The model under review builds one solid part; all positions refer to its coordinate system, in mm. A direction names the side the tool comes from. Coordinates: 2 decimals unless noted, no trailing zeros. Order: outer loops, then holes, each group sorted by start corner. A loop starts at its lowest first (then second) coordinate and runs counter-clockwise, first axis right, second up.
```python
from build123d import *

# Parameters (mm, degrees)
F0_R     = 15
F1_DEPTH = 25
F3_D     = 25.1
F3_DEPTH = 20
F3_TIP   = 7.5408007688
F5_R     = 15
F6_DEPTH = 25
F8_T     = -2
F9_D     = 2


with BuildPart() as f1:
    # F0 (on Front) → F1 (new body)
    with BuildSketch(Plane.XZ):
        Circle(F0_R)
    extrude(amount=F1_DEPTH)

    # F3
    with Locations(Plane.XZ.offset(25)):
        with Locations((0, 0)):
            Hole(F3_D / 2, depth=F3_DEPTH)
            with Locations((0, 0, -(F3_DEPTH + F3_TIP / 2))):  # 118° drill point
                Cone(0, F3_D / 2, F3_TIP, mode=Mode.SUBTRACT)


with BuildPart() as f6:
    # F5 (on Front) → F6 (new body)
    with BuildSketch(Plane.XZ):
        Circle(F5_R)
    extrude(amount=F6_DEPTH)

    # F8
    f8_openings = [f6.faces().sort_by_distance(p)[0] for p in [
        (0, -25, 0),
    ]]
    offset(amount=F8_T, openings=f8_openings)

    # F9 (through all)
    with Locations(Plane.XZ.offset(25)):
        with Locations((0, 0)):
            Hole(F9_D / 2)


solid = f6.part
```
(1) Draft analysis for pull direction Z (two halves, no side actions). For faces 3 (the face through (3, -2, 0)), 4 (the face through (-0.1, -25, 13.4)), 5 (the face through (-14.985, -12.325, 0.66)), state which applies: released by +Z, released by -Z, zero draft, split by the parting line, or undercut.
A:
face 3: undercut
face 4: zero draft
face 5: split by the parting line
(2) We need section B-B, the plane x = 0. Write out the cut boundary in (y, z), and give its area (3 significant figures).
A:
outline: (-25, -15) - (0, -15) - (0, -1) - (-2, -1) - (-2, -13) - (-25, -13) - close; (-25, 13) - (-2, 13) - (-2, 1) - (0, 1) - (0, 15) - (-25, 15) - close
area: 148 mm2
(3) We need section C-C, the plane y = -16. Write out the cut boundary in (x, z).
A:
outline: circle Ø30 at (0, 0); hole circle Ø26 at (0, 0)
(4) Machinability: for faces 1 (the face through (0, -1, -1)), 2 (the face through (-10.316, -13.339, -7.91)), which of the approach directions +Z, -Z, +X, -X, +Y, -Y give a long, thin tool a straight path to every point of the face, cutting with its end or side? Answer none if there is none.
A:
face 1: +Y, -Y
face 2: -Y
(5) Wall thickness on probe 1 along Z at (x, y) = (0, -1.25); probe 2 along X at (y, z) = (-18.25, -0.25): over which ranges is each line inside the solid? List them lowest first.
A:
probe 1: z = -15 to -1, 1 to 15
probe 2: x = -15 to -13, 13 to 15
(6) For pin 1 Ø4 at (y, z) = (-6, -3) entering from +X; pin 2 Ø8 at (x, z) = (2, 1.5) entering from -Y; pin 3 Ø4 at (y, z) = (-13, 8.5) entering from -X, all flat-tipped, find the tip position at first contact; note any pin that passes through.
A:
pin 1: stops at x = 14.97
pin 2: stops at y = -2
pin 3: stops at x = -13.52
(7) We need section A-A, the plane z = 0. Write out the cut boundary in (x, y).
A:
outline: (-15, -25) - (-13, -25) - (-13, -2) - (-1, -2) - (-1, 0) - (-15, 0) - close; (1, -2) - (13, -2) - (13, -25) - (15, -25) - (15, 0) - (1, 0) - close
(8) We need section D-D, the plane z = 6.25. Write out the cut boundary in (x, y), and give its area (3 significant figures).
A:
outline: (-13.64, -25) - (-11.4, -25) - (-11.4, -2) - (11.4, -2) - (11.4, -25) - (13.64, -25) - (13.64, 0) - (-13.64, 0) - close
area: 157 mm2
